Geometry check sheet. Reference: the model listing, model coordinates, mm. A direction names the side the tool comes from. Round coordinates to 2 decimals unless told otherwise and drop trailing zeros. Write each loop counter-clockwise with the first axis right and the second up, starting at its lowest first coordinate (ties: lowest second). Pieces come first, ordered by that corner, then holes. Notation, with made-up numbers: (-9.75, 33) -> (35.25, 33) arc R23 ccw to (35.25, 63) -> close; hole circle Ø6 at (-16, 4.5). An arc over 180 degrees is marked (long way). Return JSON: item names as keys, results as strings. Group by question number.
from build123d import *

# Parameters (mm, degrees)
BOSS_EXTRUDE1_DEPTH = 10
CUT_EXTRUDE1_DEPTH  = 7.75
SKETCH3_R           = 2.75
CUT_EXTRUDE2_DEPTH  = 15.5
SKETCH4_R           = 2.75
CUT_EXTRUDE3_DEPTH  = 15.5


with BuildPart() as part:
    # Sketch1 → Boss-Extrude1 (new, symmetric)
    with BuildSketch(Plane(origin=(0, 0, 0), x_dir=(0, 0, -1), z_dir=(1, 0, 0))):
        Polygon((-15, 0), (15, 0), (15, 30), (10.5, 30), (-15, 4.5), align=None)
    extrude(amount=BOSS_EXTRUDE1_DEPTH, both=True)

    # Sketch2 → Cut-Extrude1 (cut, symmetric)
    with BuildSketch(Plane(origin=(0, 0, 0), x_dir=(0, 0, -1), z_dir=(1, 0, 0))):
        Polygon((-11.25, 4.5), (11.25, 4.5), (11.25, 26.129344049), (11.25, 30), (10.5, 30), (-15, 4.5), align=None)
    extrude(amount=CUT_EXTRUDE1_DEPTH, both=True, mode=Mode.SUBTRACT)

    # Sketch3 → Cut-Extrude2 (cut)
    with BuildSketch(Plane.XY.offset(-11.25)):
        with Locations((0, 18)):
            Circle(SKETCH3_R)
    extrude(amount=-CUT_EXTRUDE2_DEPTH, mode=Mode.SUBTRACT)

    # Sketch4 → Cut-Extrude3 (cut)
    with BuildSketch(Plane(origin=(0, 4.5, 0), x_dir=(1, 0, 0), z_dir=(0, 1, 0))):
        with Locations(Location((0, -3, 0), (0, 0, 270))):
            Circle(SKETCH4_R)
    extrude(amount=-CUT_EXTRUDE3_DEPTH, mode=Mode.SUBTRACT)


solid = part.part
1) Go/stop test with flat-tipped pins: P1, Ø8, axis at x = -1, z = 8, coming from the +Y side; P2, Ø2, axis at x = 4.5, y = 13.5, coming from the +Z side. Record where each tip stops, or that it passes through.
2) Sectioned sample at D-D on z = -8. Enter the section's corners in (x, y), and give its area (4 significant figures).
3) Sectioned sample at B-B on y = 18. Enter the section's corners in (x, z).
4) Sectioned sample at C-C on y = 13. Enter the section's corners in (x, z).
5) Mould release check, pull along Y, two halves, no side actions. Record for faces 3 (the face through (0, 0, 0)), 4 (the face through (10, 12, -3)), 5 (the face through (-8.9, 17.4, 2.1)), 6 (the face through (-0.358, 20.727, -13.099)): +Y half, -Y half, draft (parallel to the pull), parting line (faces both ways), or undercut.
6) Material ranges on probe 1 along X at (y, z) = (6.75, 11); probe 2 along Z at (x, y) = (-5.5, 7.25); probe 3 along Y at (x, z) = (4.5, 7.5), recorded low to high. Write a range as [from, to].
7) Tool access check on faces 1 (the face through (-10, 12, -3)), 2 (the face through (0, 4.5, -1)). Record the directions out of +Z, -Z, +X, -X, +Y, -Y that give a thin tool (end or side, any length) a straight path to the whole face; none if there is none.
8) Sectioned sample at A-A on z = 3. Enter the section's corners in (x, y), and give its area (3 significant figures).
Evaluation:
{
 "1": {"P1": "stops at y = 4.5", "P2": "stops at z = -11.25"},
 "2": {"outline": "(-10, 0) -> (10, 0) -> (10, 27.5) -> (7.75, 27.5) -> (7.75, 4.5) -> (-7.75, 4.5) -> (-7.75, 27.5) -> (-10, 27.5) -> close", "area": "193.5 mm2"},
 "3": {"outline": "(-10, -15) -> (-2.75, -15) -> (-2.75, -11.25) -> (-7.75, -11.25) -> (-7.75, 1.5) -> (-10, 1.5) -> close; (2.75, -15) -> (10, -15) -> (10, 1.5) -> (7.75, 1.5) -> (7.75, -11.25) -> (2.75, -11.25) -> close"},
 "4": {"outline": "(-10, -15) -> (10, -15) -> (10, 6.5) -> (7.75, 6.5) -> (7.75, -11.25) -> (-7.75, -11.25) -> (-7.75, 6.5) -> (-10, 6.5) -> close"},
 "5": {"face 3": "-Y half", "face 4": "draft", "face 5": "+Y half", "face 6": "undercut"},
 "6": {"probe 1": "x = [-10, -7.75], [7.75, 10]", "probe 2": "z = [-15, -11.25]", "probe 3": "y = [0, 4.5]"},
 "7": {"face 1": "+Z, -Z, -X, +Y, -Y", "face 2": "+Z, +Y"},
 "8": {"outline": "(-10, 0) -> (-2.75, 0) -> (-2.75, 4.5) -> (-7.75, 4.5) -> (-7.75, 16.5) -> (-10, 16.5) -> close; (2.75, 0) -> (10, 0) -> (10, 16.5) -> (7.75, 16.5) -> (7.75, 4.5) -> (2.75, 4.5) -> close", "area": "119 mm2"}
}
